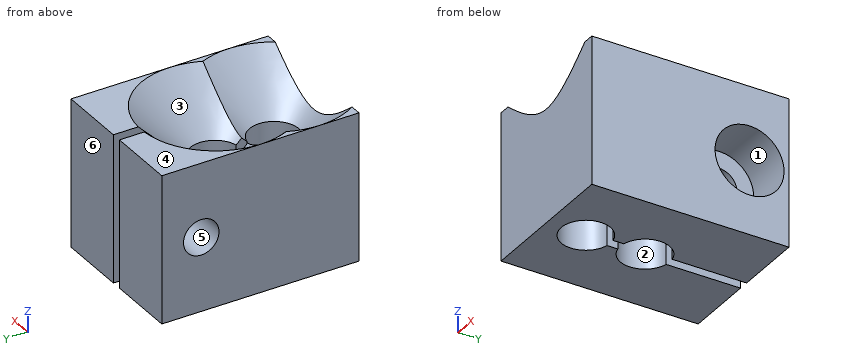
from build123d import *

# Parameters (mm, degrees)
SZKIC1_W                                             = 15
SZKIC1_H                                             = 15
DODANIE_WYCI_GNI_CIE1_DEPTH                          = 20
POG_BIENIE_WALCOWE_POD_M3_WKR_T_DO_CZ_CI_D           = 3.6
POG_BIENIE_WALCOWE_POD_M3_WKR_T_DO_CZ_CI_CBORE_D     = 7
POG_BIENIE_WALCOWE_POD_M3_WKR_T_DO_CZ_CI_CBORE_DEPTH = 5
POG_BIENIE_STO_KOWE_POD_M5_WKR_T_DO_CZ_C_D           = 5
POG_BIENIE_STO_KOWE_POD_M5_WKR_T_DO_CZ_C_CSINK_D     = 15
POG_BIENIE_STO_KOWE_POD_M5_WKR_T_DO_CZ_C_CSINK_ANGLE = 90
SZKIC3_W                                             = 1
SZKIC3_H                                             = 13.577845222
WYTNIJ_WYCI_GNI_CIE1_DEPTH                           = 16


with BuildPart() as part:
    # Szkic1 → Dodanie-wyci_gni_cie1 (new body)
    with BuildSketch(Plane(origin=(0, 0, 0), x_dir=(1, 0, 0), z_dir=(0, 1, 0))):
        Rectangle(SZKIC1_W, SZKIC1_H)
    extrude(amount=DODANIE_WYCI_GNI_CIE1_DEPTH)

    # Pog_bienie walcowe pod M3 wkr_t do cz_ci (through all)
    with Locations(Plane(origin=(7.5, 0, 0), x_dir=(0, 0, -1), z_dir=(1, 0, 0))):
        with Locations((0, 16)):
            CounterBoreHole(POG_BIENIE_WALCOWE_POD_M3_WKR_T_DO_CZ_CI_D / 2, POG_BIENIE_WALCOWE_POD_M3_WKR_T_DO_CZ_CI_CBORE_D / 2, POG_BIENIE_WALCOWE_POD_M3_WKR_T_DO_CZ_CI_CBORE_DEPTH)

    # Pog_bienie sto_kowe pod M5 wkr_t do cz_c (through all)
    with Locations(Plane.XY.offset(7.5)):
        with Locations((0, 10), (0, 4)):
            CounterSinkHole(POG_BIENIE_STO_KOWE_POD_M5_WKR_T_DO_CZ_C_D / 2, POG_BIENIE_STO_KOWE_POD_M5_WKR_T_DO_CZ_C_CSINK_D / 2, counter_sink_angle=POG_BIENIE_STO_KOWE_POD_M5_WKR_T_DO_CZ_C_CSINK_ANGLE)

    # Szkic3 → Wytnij-wyci_gni_cie1 (cut, through all)
    with BuildSketch(Plane.XY.offset(7.5)):
        with Locations((0, 13.211077389)):
            Rectangle(SZKIC3_W, SZKIC3_H)
    extrude(amount=-WYTNIJ_WYCI_GNI_CIE1_DEPTH, mode=Mode.SUBTRACT)


solid = part.part
Source: CAD feature listing. Evaluate the final solid. Frame: model axes, mm. Face numbers are marked on the shaded views. A direction names the side the tool comes from. Coordinates: 2 decimals unless noted, no trailing zeros. Order: outer loops, then holes, each group sorted by start corner. A loop starts at its lowest first (then second) coordinate and runs counter-clockwise, first axis right, second up. Notation, with made-up numbers: M -14.5,29.5 L 24.5,29.5 A10 ccw 24.5,33.5 Z; hole C 4,47 d6. An arc over 180 degrees is marked long. Write each question's results on one line, items separated by ' | '. Start each with the question number.
1. Material intervals for L1, parallel to Y at x = -2, z = -2; L2, parallel to X at y = 13, z = 0.25; L3, parallel to Y at x = -4.5, z = 0, sorted ascending.
2. Draft query along Y for the marked faces 4, 5 and 6. Return one class per face: +Y half, -Y half, draft (parallel to the pull), parting line (faces both ways), or undercut.
3. Section C-C, the plane x = 2.25. State how many separate pieces and enclosed holes the cut face has, then the cut area to 3 significant figures.
4. Pin query (flat end, axial travel): pin 1 (4 mm diameter, centred on x = -3.5, y = 5, fed in from +Z); pin 2 (2 mm diameter, centred on y = 16, z = 0, fed in from +X). Return the tip coordinate at first contact, or that it passes through.
5. Reachability of the marked faces 1, 2 and 3 from +Z, -Z, +X, -X, +Y, -Y: full face, straight path, thin tool, end or side. Return the list, or none.
6. Section A-A, the plane z = 0. Return the cut outline in (x, y), then the cut area to 3 significant figures.
7. Section B-B, the plane z = 4.75. Return the cut outline in (x, y), then the cut area to 3 significant figures.
Solution:
1) L1: 0 to 2.5, 5.5 to 8.5, 11.5 to 20 | L2: -7.5 to -0.5, 0.5 to 2.5 | L3: 0 to 14.2, 17.8 to 20
2) face 4: draft | face 5: undercut | face 6: +Y half
3) separate pieces: 3 | enclosed holes: 1 | area: 179 mm²
4) pin 1: z = 5.64 | pin 2: through
5) face 1: +X | face 2: +Z, -Z | face 3: +Z
6) outline: M -7.5,0 L 7.5,0 L 7.5,12.5 L 2.5,12.5 L 2.5,14.2 L 0.5,14.2 L 0.5,12.45 A2.5 cw 0.5,7.55 L 0.5,6.45 A2.5 cw long -0.5,6.45 L -0.5,7.55 A2.5 cw -0.5,12.45 L -0.5,14.2 L -7.5,14.2 Z; M -7.5,17.8 L -0.5,17.8 L -0.5,20 L -7.5,20 Z; M 0.5,17.8 L 2.5,17.8 L 2.5,19.5 L 7.5,19.5 L 7.5,20 L 0.5,20 Z | area: 185 mm²
7) outline: M -7.5,0 L -2.56,0 A4.75 cw -3.68,7 A4.75 cw -0.5,14.72 L -0.5,20 L -7.5,20 Z; M 0.5,14.72 A4.75 cw 3.68,7 A4.75 cw 2.56,0 L 7.5,0 L 7.5,20 L 0.5,20 Z | area: 174 mm²
